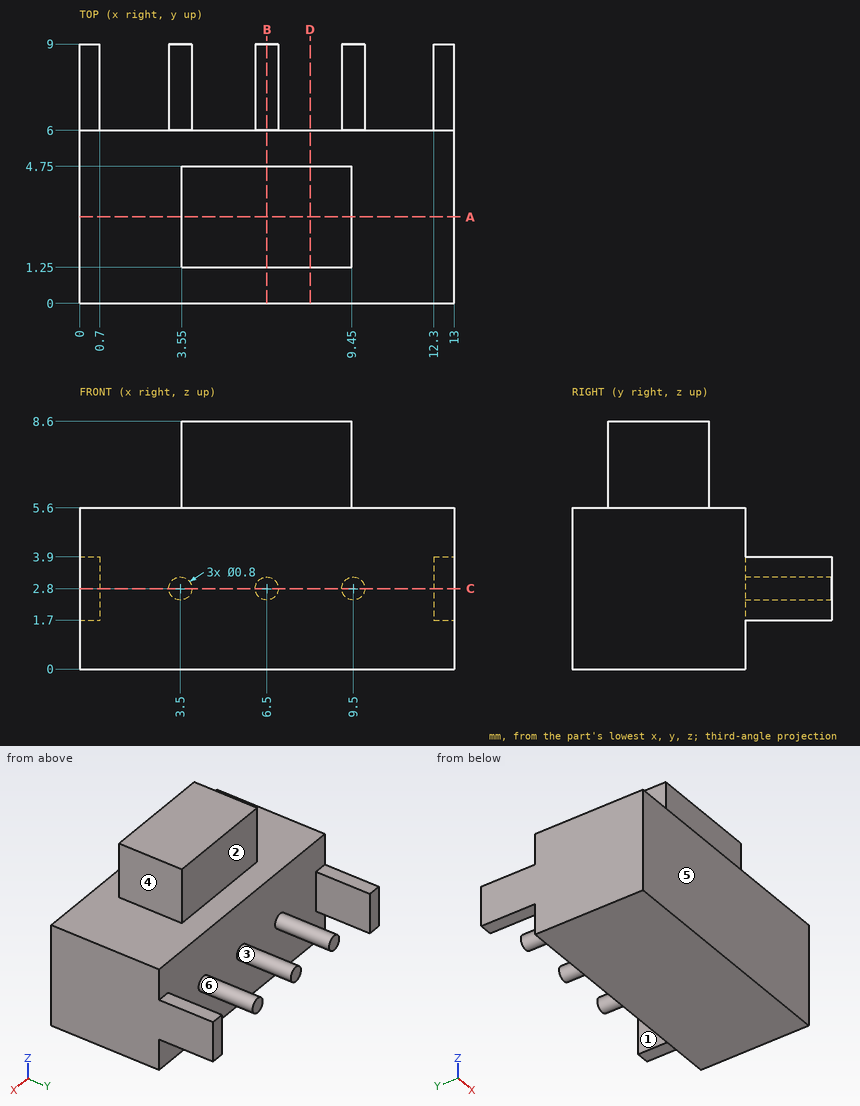
Here's the drawing with two shaded views (mm, measured from the low corner). I have some questions. A direction names the side the tool comes from. Round coordinates to 2 decimals unless told otherwise and drop trailing zeros. Loops run counter-clockwise (first coordinate to the right, second up) from the corner with the lowest first, then second, coordinate; pieces in that order, holes last. Notation, with made-up numbers: (-13, -19) - (-5, -19) arc R24 ccw to (-5, 8) - close; hole circle Ø6 at (-3, 65). An arc over 180 degrees is marked (long way). Use CSV: the item, a comma, the result in double quotes.
Item 1: Will these pins go through, and if not, where does the flat tip stop? pin 1 (1.8 mm diameter, centred on y = 8, z = 2.5, fed in from -X); pin 2 (0.8 mm diameter, centred on x = 13, y = 8, fed in from -Z); pin 3 (0.6 mm diameter, centred on x = 0.5, y = 7, fed in from +Z); pin 4 (1.5 mm diameter, centred on x = 7.5, y = 7.5, fed in from +Z).
Here are the results:
pin 1,"stops at x = 0"
pin 2,"stops at z = 1.7"
pin 3,"stops at z = 3.9"
pin 4,"stops at z = 3.11"
Item 2: If we section it at D-D on x = 8: List the corners of the cut face in (y, z) for me, then the cut area to 3 significant figures.
Here are the results:
outline,"(0, 0) - (6, 0) - (6, 5.6) - (4.75, 5.6) - (4.75, 8.6) - (1.25, 8.6) - (1.25, 5.6) - (0, 5.6) - close"
area,"44.1 mm²"
Item 3: For the marked faces 1, 2 and 3, which set-ups out of +Z, -Z, +X, -X, +Y, -Y let a thin tool reach every point of the face, with its end or its side?
Here are the results:
face 1,"+Z, -Z, +Y"
face 2,"+Z, +X, -X, +Y"
face 3,"+Y"
Item 4: If we mould it in two halves opening along X, with no side actions, what happens to the marked faces 4, 5 and 6? For each: pulls with the +X half, pulls with the -X half, needs draft (parallel to the pull), parting line crosses it, or undercut.
Here are the results:
face 4,"pulls with the +X half"
face 5,"needs draft"
face 6,"undercut"
Item 5: If we section it at B-B on x = 6.5: List the corners of the cut face in (y, z) for me, then the cut area to 3 significant figures.
Here are the results:
outline,"(0, 0) - (6, 0) - (6, 2.4) - (9, 2.4) - (9, 3.2) - (6, 3.2) - (6, 5.6) - (4.75, 5.6) - (4.75, 8.6) - (1.25, 8.6) - (1.25, 5.6) - (0, 5.6) - close"
area,"46.5 mm²"
Item 6: If we section it at A-A on y = 3: List the corners of the cut face in (x, z) for me.
Here are the results:
outline,"(0, 0) - (13, 0) - (13, 5.6) - (9.45, 5.6) - (9.45, 8.6) - (3.55, 8.6) - (3.55, 5.6) - (0, 5.6) - close"
Item 7: I need wall thicknesses on L1, parallel to Y at x = 5.75, z = 3.5; L2, parallel to Z at x = 1, y = 2.5; L3, parallel to Y at x = 8, z = 6.75. Which ranges of each line are inside material? Lowest first, please. Write a range as [from, to].
Here are the results:
L1,"y = [0, 6]"
L2,"z = [0, 5.6]"
L3,"y = [1.25, 4.75]"
Item 8: If we section it at C-C on z = 2.8: List the corners of the cut face in (x, y) for me, then the cut area to 3 significant figures.
Here are the results:
outline,"(0, 0) - (13, 0) - (13, 9) - (12.3, 9) - (12.3, 6) - (9.9, 6) - (9.9, 9) - (9.1, 9) - (9.1, 6) - (6.9, 6) - (6.9, 9) - (6.1, 9) - (6.1, 6) - (3.9, 6) - (3.9, 9) - (3.1, 9) - (3.1, 6) - (0.7, 6) - (0.7, 9) - (0, 9) - close"
area,"89.4 mm²"
